Could you check a few things on this drawing? It's one solid part, dimensions in mm from its lowest x, y, z. A direction names the side the tool comes from. Give positions to 0.01 mm unless a question says otherwise; leave off trailing zeros. Loops run counter-clockwise (first coordinate to the right, second up) from the corner with the lowest first, then second, coordinate; pieces in that order, holes last. Notation, with made-up numbers: (31.25, -31) - (90.25, -31) arc R17 cw to (90.25, -14) - close; hole circle Ø7 at (50, 67). An arc over 180 degrees is marked (long way). One line per item, written item: value. Start each with the question number.
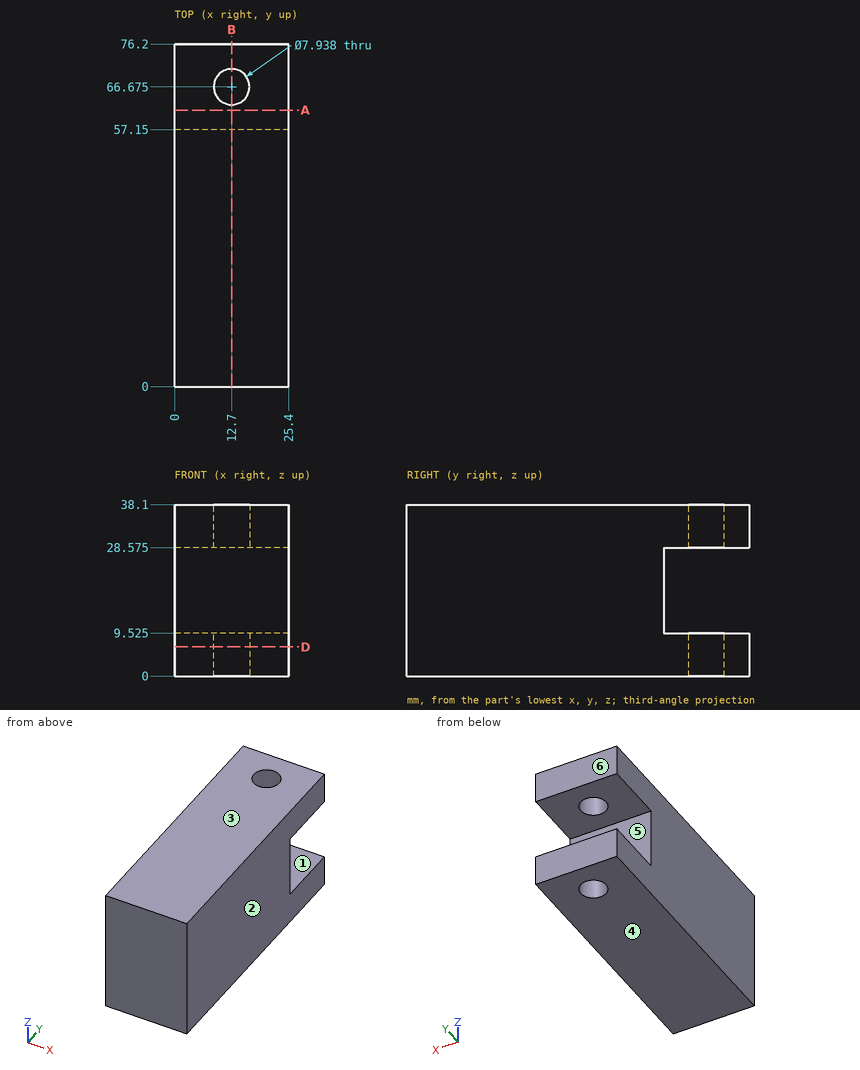
(1) If we mould it in two halves opening along Z, with no side actions, what happens to the marked faces 1, 2, 3 and 4? For each: pulls with the +Z half, pulls with the -Z half, needs draft (parallel to the pull), parting line crosses it, or undercut.
(2) If we section it at A-A on y = 61.5: List the corners of the cut face in (x, z) for me (1 decimal), plus the area to 3 significant figures.
(3) For the marked faces 5 and 6, which set-ups out of +Z, -Z, +X, -X, +Y, -Y let a thin tool reach every point of the face, with its end or its side?
(4) Will this pin go through, and if not, where does the flat tip stop? pin 1 (12 mm diameter, centred on x = 4, z = 19.5, fed in from +Y).
(5) If we section it at D-D on z = 6.5: List the corners of the cut face in (x, y) for me (1 decimal), plus the area to 3 significant figures.
(6) If we section it at B-B on x = 12.7: Give the number of separate pieces and of enclosed holes in the cut face, plus the area to 3 significant figures.
(7) Please list where these lines run through material, in increasing order: probe 1 along Z at (x, y) = (18, 62) (1 decimal); probe 2 along Y at (x, z) = (12.7, 32); probe 3 along Y at (x, z) = (1, 15). Write a range as from..to.
Found:
1. face 1: undercut
1. face 2: needs draft
1. face 3: pulls with the +Z half
1. face 4: pulls with the -Z half
2. outline: (0, 0) - (25.4, 0) - (25.4, 9.5) - (0, 9.5) - close; (0, 28.6) - (25.4, 28.6) - (25.4, 38.1) - (0, 38.1) - close
2. area: 484 mm^2
3. face 5: +X, -X, +Y
3. face 6: +Z, -Z, +X, -X, +Y
4. pin 1: y = 57.15
5. outline: (0, 0) - (25.4, 0) - (25.4, 76.2) - (0, 76.2) - close; hole circle Ø7.9 at (12.7, 66.7)
5. area: 1,890 mm^2
6. separate pieces: 3
6. enclosed holes: 0
6. area: 2,390 mm^2
7. probe 1: 0..9.5, 28.6..38.1
7. probe 2: 0..62.71, 70.64..76.2
7. probe 3: 0..57.15
